Answer from the drawing. Dimensions are ordinates in mm from the lowest x, y and z of the part. A direction names the side the tool comes from. Round coordinates to 2 decimals unless told otherwise and drop trailing zeros. Write each loop counter-clockwise with the first axis right and the second up, starting at its lowest first coordinate (ties: lowest second). Pieces come first, ordered by that corner, then holes. Notation, with made-up numbers: (67, 50) - (105, 50) arc R19 ccw to (105, 78) - close; hole circle Ø4 at (60.25, 79.5). An arc over 180 degrees is marked (long way). Answer in a Markdown table with one row per item.
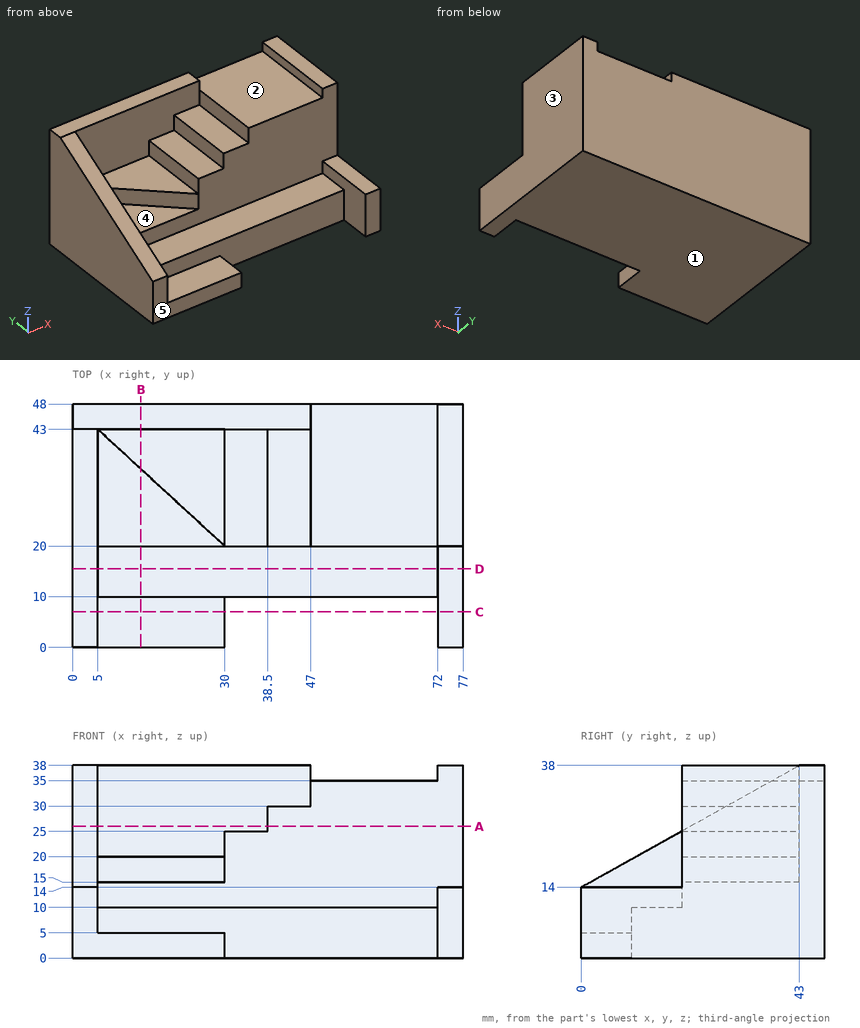
(1) Section C-C (y = 7) is taken. Give the vertices of the cut face in (x, z).
Checked values:
| item | result |
|---|---|
| outline | (0, 0) - (30, 0) - (30, 5) - (5, 5) - (5, 17.91) - (0, 17.91) - close; (72, 0) - (77, 0) - (77, 14) - (72, 14) - close |
(2) Section A-A (z = 26) is taken. Give the vertices of the cut face in (x, y).
Checked values:
| item | result |
|---|---|
| outline | (0, 21.5) - (5, 21.5) - (5, 43) - (38.5, 43) - (38.5, 20) - (77, 20) - (77, 48) - (0, 48) - close |
(3) Section D-D (y = 15.5) is taken. Give the vertices of the cut face in (x, z).
Checked values:
| item | result |
|---|---|
| outline | (0, 0) - (77, 0) - (77, 14) - (72, 14) - (72, 10) - (5, 10) - (5, 22.65) - (0, 22.65) - close |
(4) Flat-ended cylindrical pins translate along their axes: pin 1 (3.5 mm diameter, centred on y = 34.5, z = 37, fed in from -X); pin 2 (5.5 mm diameter, centred on x = 16.5, z = 27.5, fed in from -Y); pin 3 (4 mm diameter, centred on x = 43.5, y = 33, fed in from +Z). Find the tip coordinate at first contact, or state that the pin passes through.
Checked values:
| item | result |
|---|---|
| pin 1 | stops at x = 72 |
| pin 2 | stops at y = 43 |
| pin 3 | stops at z = 30 |
(5) Find the intervals of material crossed by line 1 (Z direction, x = 15, y = 22); line 2 (Y direction, x = 62, z = 12.5); line 3 (Z direction, x = 27, y = 29), in increasing order.
Checked values:
| item | result |
|---|---|
| line 1 | z = 0 to 15 |
| line 2 | y = 20 to 48 |
| line 3 | z = 0 to 20 |
(6) Section B-B (x = 13.5) is taken. Give the vertices of the cut face in (y, z).
Checked values:
| item | result |
|---|---|
| outline | (0, 0) - (48, 0) - (48, 38) - (43, 38) - (43, 20) - (35.18, 20) - (35.18, 15) - (20, 15) - (20, 10) - (10, 10) - (10, 5) - (0, 5) - close |
(7) For a pull along X with two mould halves and no side action, classify the marked faces 1, 2 and 3 as pulls with the +X half, pulls with the -X half, needs draft (parallel to the pull), parting line crosses it, or undercut.
Checked values:
| item | result |
|---|---|
| face 1 | needs draft |
| face 2 | undercut |
| face 3 | pulls with the +X half |
(8) For the marked faces 4 and 5, determine the directions among +Z, -Z, +X, -X, +Y, -Y from which every point of the face is accessible in a straight line to the end or side of a thin tool.
Checked values:
| item | result |
|---|---|
| face 4 | +Z, -Y |
| face 5 | +Z, -Z, +X, -X, -Y |
